Geometry check sheet. Reference: the model listing, model coordinates, mm. A direction names the side the tool comes from. Coordinates: 2 decimals unless noted, no trailing zeros. Write each loop counter-clockwise with the first axis right and the second up, starting at its lowest first coordinate (ties: lowest second). Pieces come first, ordered by that corner, then holes. Notation, with made-up numbers: (-29, -26.75) -> (-1, -26.75) arc R23 ccw to (-1, -7.75) -> close; hole circle Ø1 at (-5, 5). An arc over 180 degrees is marked (long way). Answer in a Markdown table with one row per item. Add a question column.
Q1. Tool access check on faces 1 (the face through (5.347, 10.619, 0.018)), 2 (the face through (-12.842, 1.237, 2.773)). Record the directions out of +Z, -Z, +X, -X, +Y, -Y that give a thin tool (end or side, any length) a straight path to the whole face; none if there is none.
Q2. Gauge pin test, flat end, axial feed: P1, Ø5.5, axis at x = 0, y = 7.02, coming from the -Z side. Record the tip position at first contact, or that the pin passes through.
Q3. Section check A-A, the plane x = 0. Record the boundary of the cut face in (y, z), and give its area (3 significant figures).
Q4. Thickness scan on line 1 (Z direction, x = -9, y = 6.5); line 2 (Y direction, x = 0, z = -1.65). Record the ranges inside material, lowest first.
```python
from build123d import *

# Parameters (mm, degrees)
F1_DEPTH = 1.25
F2_T     = 2
F3_R     = 2.38125
F4_DEPTH = 6.501
F6_DEPTH = 3.25
F7_SIZE  = 5.08
F8_R     = 5.08
F9_R     = 1.5875
F10_SIZE = 0.79375
F11_R    = 0.79375


with BuildPart() as f1:
    # F0 (on Top) → F1 (new body, symmetric)
    with BuildSketch(Plane.XY):
        with BuildLine():
            ThreePointArc((1.2815576559, 11.8657501741), (0, 12.1358861541), (-1.2815576559, 11.8657501741))
            Line((-1.2815576559, 11.8657501741), (-8.9015576559, 8.5039854683))
            ThreePointArc((-8.9015576559, 8.5039854683), (-10.2798468525, 7.3328572186), (-10.795, 5.5991214483))
            Line((-10.795, 5.5991214483), (-10.795, -5.5991214483))
            Line((-10.795, -5.5991214483), (10.795, -5.5991214483))
            Line((10.795, -5.5991214483), (10.795, 5.5991214483))
            ThreePointArc((10.795, 5.5991214483), (10.2798468525, 7.3328572186), (8.9015576559, 8.5039854683))
            Line((8.9015576559, 8.5039854683), (1.2815576559, 11.8657501741))
        make_face()
        with BuildLine():
            Line((-8.9015576559, 8.5039854683), (-1.2815576559, 11.8657501741))
            ThreePointArc((-1.2815576559, 11.8657501741), (0, 12.1358861541), (1.2815576559, 11.8657501741))
            Line((1.2815576559, 11.8657501741), (8.9015576559, 8.5039854683))
            ThreePointArc((8.9015576559, 8.5039854683), (10.2798468525, 7.3328572186), (10.795, 5.5991214483))
            Line((10.795, 5.5991214483), (10.795, -5.5991214483))
            Line((10.795, -5.5991214483), (11.295, -5.5991214483))
            Line((11.295, -5.5991214483), (11.295, 5.5991214483))
            ThreePointArc((11.295, 5.5991214483), (10.6987203726, 7.6058864738), (9.1033777592, 8.961444369))
            Line((9.1033777592, 8.961444369), (1.4833777592, 12.3232090749))
            ThreePointArc((1.4833777592, 12.3232090749), (0, 12.6358861541), (-1.4833777592, 12.3232090749))
            Line((-1.4833777592, 12.3232090749), (-9.1033777592, 8.961444369))
            ThreePointArc((-9.1033777592, 8.961444369), (-10.6987203726, 7.6058864738), (-11.295, 5.5991214483))
            Line((-11.295, 5.5991214483), (-11.295, -5.5991214483))
            Line((-11.295, -5.5991214483), (-10.795, -5.5991214483))
            Line((-10.795, -5.5991214483), (-10.795, 5.5991214483))
            ThreePointArc((-10.795, 5.5991214483), (-10.2798468525, 7.3328572186), (-8.9015576559, 8.5039854683))
        make_face()
    extrude(amount=F1_DEPTH, both=True)

    # F2
    f2_openings = [f1.faces().sort_by_distance(p)[0] for p in [
        (0, -5.599121, 0),
    ]]
    offset(amount=F2_T, openings=f2_openings, kind=Kind.INTERSECTION)

    # F3 (on face) → F4 (cut, through all)
    with BuildSketch(Plane(origin=(0, 0, -3.25), x_dir=(1, 0, 0), z_dir=(0, 0, -1))):
        with Locations((0, -7.0158861541)):
            Circle(F3_R)
    extrude(amount=-F4_DEPTH, mode=Mode.SUBTRACT)

    # F5 (on Top) → F6 (join, symmetric)
    with BuildSketch(Plane.XY):
        with BuildLine():
            Line((-9.9106581723, 10.7912799722), (-2.2906581723, 14.1530446781))
            ThreePointArc((-2.2906581723, 14.1530446781), (-1.1704967699, 14.5138639419), (0, 14.6358861541))
            Line((0, 14.6358861541), (-13.295, 14.6358861541))
            Line((-13.295, 14.6358861541), (-13.295, 5.5991214483))
            ThreePointArc((-13.295, 5.5991214483), (-12.3742144529, 8.6980034944), (-9.9106581723, 10.7912799722))
        make_face()
        with BuildLine():
            Line((13.295, 14.6358861541), (0, 14.6358861541))
            ThreePointArc((0, 14.6358861541), (1.1704967699, 14.5138639419), (2.2906581723, 14.1530446781))
            Line((2.2906581723, 14.1530446781), (9.9106581723, 10.7912799722))
            ThreePointArc((9.9106581723, 10.7912799722), (12.3742144529, 8.6980034944), (13.295, 5.5991214483))
            Line((13.295, 5.5991214483), (13.295, 14.6358861541))
        make_face()
    extrude(amount=F6_DEPTH, both=True)

    # F7
    f7_edges = [f1.edges().sort_by_distance(p)[0] for p in [
        (-13.295, 14.635886, 0),
        (13.295, 14.635886, 0),
    ]]
    chamfer(f7_edges, length=F7_SIZE)

    # F8
    f8_edges = [f1.edges().sort_by_distance(p)[0] for p in [
        (-13.295, 9.555886, 0),
        (13.295, 9.555886, 0),
    ]]
    fillet(f8_edges, radius=F8_R)

    # F9
    f9_edges = [f1.edges().sort_by_distance(p)[0] for p in [
        (-13.295, 0.92628, -3.25),
        (-13.295, 0.92628, 3.25),
        (13.295, 0.92628, 3.25),
        (13.295, 0.92628, -3.25),
        (12.908308, 9.395713, -3.25),
        (10.011051, 12.839835, -3.25),
        (-12.908308, 9.395713, -3.25),
        (-10.011051, 12.839835, -3.25),
        (12.908308, 9.395713, 3.25),
        (10.011051, 12.839835, 3.25),
        (-12.908308, 9.395713, 3.25),
        (-10.011051, 12.839835, 3.25),
    ]]
    fillet(f9_edges, radius=F9_R)

    # F10
    f10_edges = [f1.edges().sort_by_distance(p)[0] for p in [
        (-2.38125, 7.015886, -3.25),
        (-2.38125, 7.015886, 3.25),
    ]]
    chamfer(f10_edges, length=F10_SIZE)

    # F11
    f11_edges = [f1.edges().sort_by_distance(p)[0] for p in [
        (0, -5.599121, -3.25),
        (0, -5.599121, 3.25),
        (12.830032, -5.599121, 2.785032),
        (-12.830032, -5.599121, 2.785032),
        (13.295, -5.599121, 0),
        (-13.295, -5.599121, 0),
        (12.830032, -5.599121, -2.785032),
        (-12.830032, -5.599121, -2.785032),
    ]]
    fillet(f11_edges, radius=F11_R)


solid = f1.part
```
Calculated:
| question | item | result |
|---|---|---|
| 1 | face 1 | -Y |
| 1 | face 2 | +Z, -X, +Y, -Y |
| 2 | P1 | stops at z = -2.83 |
| 3 | outline | (-5.6, -2.46) arc R0.79 ccw to (-4.81, -3.25) -> (3.84, -3.25) -> (4.63, -2.46) -> (4.63, -1.25) -> (-5.6, -1.25) -> close; (-5.6, 1.25) -> (4.63, 1.25) -> (4.63, 2.46) -> (3.84, 3.25) -> (-4.81, 3.25) arc R0.79 ccw to (-5.6, 2.46) -> close; (9.4, -2.46) -> (10.19, -3.25) -> (14.64, -3.25) -> (14.64, 3.25) -> (10.19, 3.25) -> (9.4, 2.46) -> (9.4, 1.25) -> (12.64, 1.25) -> (12.64, -1.25) -> (9.4, -1.25) -> close |
| 3 | area | 65.4 mm² |
| 4 | line 1 | z = -3.25 to -1.25, 1.25 to 3.25 |
| 4 | line 2 | y = -5.6 to 4.63, 9.4 to 14.64 |
